The model under review builds one solid part; all positions refer to its coordinate system, in mm. A direction names the side the tool comes from. Round coordinates to 2 decimals unless told otherwise and drop trailing zeros. Order: outer loops, then holes, each group sorted by start corner. A loop starts at its lowest first (then second) coordinate and runs counter-clockwise, first axis right, second up.
1) Consider section B-B (x = 0). Give the boundary of the cut face in (y, z).
2) Consider section A-A (y = -5). Give the boundary of the cut face in (x, z).
3) Consider section D-D (y = 19). Give the boundary of the cut face in (x, z), then the cut area to 3 significant figures.
4) Mouldability with a two-part tool opening along Z and no side actions: class faces 1 (the face through (-9.5, 5.9, 0)), 2 (the face through (18.3, 7.5, 6.3)), 3 (the face through (19, 2.5, 5)) as pulls with the +Z half, pulls with the -Z half, needs draft (parallel to the pull), parting line crosses it, or undercut.
5) Machinability: for faces 4 (the face through (17, -10, 3)), 5 (the face through (-33, -9.998, 5)), 6 (the face through (-33, 9.998, 5)), which of the approach directions +Z, -Z, +X, -X, +Y, -Y give a long, thin tool a straight path to every point of the face, cutting with its end or side? Answer none if there is none.
6) Consider section C-C (x = 17). Give the boundary of the cut face in (y, z).
7) To check wall thickness, follow L1, parallel to Y at x = 0, z = 8.5; L2, parallel to Z at x = 17, y = 5; L3, parallel to X at y = -0.5, z = 1. State the ranges of each line that lie inside material, in increasing order.
8) Clearance check with flat-ended pins moving along their axes: P1, Ø1.8, axis at x = 17, z = 5, coming from the -Y side; P2, Ø3, axis at x = 18.5, z = 4, coming from the -Y side; P3, Ø1.5, axis at y = 1, z = 1.5, coming from the +X side; P4, Ø3, axis at y = -5, z = 5.5, coming from the +X side. State where each tip first meets the part, or that it passes through.
from build123d import *

# Parameters (mm, degrees)
SKETCH1_R               = 25
SKETCH1_R_2             = 11
BOSS_EXTRUDE1_DEPTH     = 10
CUT_EXTRUDE1_DEPTH      = 10
SKETCH5_R               = 1.5
CUT_EXTRUDE4_DEPTH      = 28.5
CUT_EXTRUDE4_DEPTH_BACK = 23.5
CUT_EXTRUDE5_START      = 30
SKETCH6_R               = 3
CUT_EXTRUDE5_DEPTH      = 20
CUT_EXTRUDE6_START      = -30
CUT_EXTRUDE6_DEPTH      = 25
CUT_EXTRUDE8_START      = 20
SKETCH8_R               = 3
CUT_EXTRUDE8_DEPTH      = 15
SKETCH9_W               = 20
SKETCH9_H               = 19.995459106
SKETCH9_R               = 1.5
BOSS_EXTRUDE2_DEPTH     = 10


with BuildPart() as part:
    # Sketch1 → Boss-Extrude1 (new body)
    with BuildSketch(Plane.XY):
        Circle(SKETCH1_R)
        Circle(SKETCH1_R_2, mode=Mode.SUBTRACT)
    extrude(amount=BOSS_EXTRUDE1_DEPTH)

    # Sketch2 → Cut-Extrude1 (cut)
    with BuildSketch(Plane.XY.offset(10)):
        Polygon((25, 0), (25, 2.5), (0, 2.5), (0, 0), (0, -2.5), (25, -2.5), align=None)
    extrude(amount=-CUT_EXTRUDE1_DEPTH, mode=Mode.SUBTRACT)

    # Sketch5 → Cut-Extrude4 (cut, two sides)
    with BuildSketch(Plane(origin=(0, -2.5, 0), x_dir=(1, 0, 0), z_dir=(0, 1, 0))) as cut_extrude4_sk:
        with Locations((17, -5)):
            Circle(SKETCH5_R)
    extrude(amount=CUT_EXTRUDE4_DEPTH, mode=Mode.SUBTRACT)
    extrude(cut_extrude4_sk.sketch, amount=-CUT_EXTRUDE4_DEPTH_BACK, mode=Mode.SUBTRACT)

    # Sketch6 → Cut-Extrude5 (cut)
    with BuildSketch(Plane(origin=(0, -2.5, 0), x_dir=(1, 0, 0), z_dir=(0, 1, 0)).offset(CUT_EXTRUDE5_START)):
        with Locations((17, -5)):
            Circle(SKETCH6_R)
    extrude(amount=-CUT_EXTRUDE5_DEPTH, mode=Mode.SUBTRACT)

    # Sketch7 → Cut-Extrude6 (cut)
    with BuildSketch(Plane(origin=(0, -2.5, 0), x_dir=(1, 0, 0), z_dir=(0, 1, 0)).offset(CUT_EXTRUDE6_START)):
        Polygon((19.309401077, -5), (18.154700538, -3), (15.845299462, -3), (14.690598923, -5), (15.845299462, -7), (18.154700538, -7), align=None)
    extrude(amount=CUT_EXTRUDE6_DEPTH, mode=Mode.SUBTRACT)

    # Sketch8 → Cut-Extrude8 (cut)
    with BuildSketch(Plane.XZ.offset(7.5).offset(CUT_EXTRUDE8_START)):
        with Locations((17, 5)):
            Circle(SKETCH8_R)
    extrude(amount=-CUT_EXTRUDE8_DEPTH, mode=Mode.SUBTRACT)

    # Sketch9 → Boss-Extrude2 (add)
    with BuildSketch(Plane(origin=(0, 0, 0), x_dir=(-1, 0, 0), z_dir=(0, 0, -1))):
        with Locations((32.913869245, 0)):
            Rectangle(SKETCH9_W, SKETCH9_H)
        with Locations((32.913869245, 5)):
            Circle(SKETCH9_R, mode=Mode.SUBTRACT)
        with Locations((32.913869245, -5)):
            Circle(SKETCH9_R, mode=Mode.SUBTRACT)
    extrude(amount=-BOSS_EXTRUDE2_DEPTH)


solid = part.part
Answer below:
1. outline: (-25, 0) - (-11, 0) - (-11, 10) - (-25, 10) - close; (11, 0) - (25, 0) - (25, 10) - (11, 10) - close
2. outline: (-42.91, 0) - (-34.41, 0) - (-34.41, 10) - (-42.91, 10) - close; (-31.41, 0) - (-9.8, 0) - (-9.8, 10) - (-31.41, 10) - close; (9.8, 0) - (24.49, 0) - (24.49, 10) - (9.8, 10) - close; hole circle Ø3 at (17, 5)
3. outline: (-16.25, 0) - (16.25, 0) - (16.25, 2.1) arc R3 cw to (16.25, 7.9) - (16.25, 10) - (-16.25, 10) - close
3. area: 315 mm2
4. face 1: pulls with the -Z half
4. face 2: undercut
4. face 3: needs draft
5. face 4: -Y
5. face 5: +Z, -Z, -X, -Y
5. face 6: +Z, -Z, -X, +Y
6. outline: (-18.33, 0) - (-2.5, 0) - (-2.5, 3.5) - (-7.5, 3.5) - (-7.5, 3) - (-12.5, 3) - (-12.5, 2) - (-18.33, 2) - close; (-18.33, 8) - (-12.5, 8) - (-12.5, 7) - (-7.5, 7) - (-7.5, 6.5) - (-2.5, 6.5) - (-2.5, 10) - (-18.33, 10) - close; (2.5, 0) - (18.33, 0) - (18.33, 2) - (7.5, 2) - (7.5, 3.5) - (2.5, 3.5) - close; (2.5, 6.5) - (7.5, 6.5) - (7.5, 8) - (18.33, 8) - (18.33, 10) - (2.5, 10) - close
7. L1: y = -25 to -11, 11 to 25
7. L2: z = 0 to 3.5, 6.5 to 10
7. L3: x = -42.91 to -10.99
8. P1: passes through
8. P2: stops at y = -16.62
8. P3: stops at x = -10.86
8. P4: stops at x = 24.75
